Build history of the part. All positions in model axes, mm. Face numbers are marked on the shaded views. A direction names the side the tool comes from. Round coordinates to 2 decimals unless told otherwise and drop trailing zeros. Write each loop counter-clockwise with the first axis right and the second up, starting at its lowest first coordinate (ties: lowest second). Pieces come first, ordered by that corner, then holes. Notation, with made-up numbers: (0, 40) - (51, 40) arc R20 cw to (51, 47) - close; hole circle Ø2 at (-19.75, 87). An arc over 180 degrees is marked (long way). Answer as a JSON object with one key per item and string values. Group by question number.
Item 1: Slice it at A-A, the plane z = 3. List the corners of the cut face in (x, y).
Item 2: Flat gauge pins, fed straight in: pin 1 (6 mm diameter, centred on y = 5.5, z = 1.5, fed in from +X); pin 2 (3.5 mm diameter, centred on x = 6.5, y = 3.5, fed in from -Z); pin 3 (1.6 mm diameter, centred on x = 56.5, y = 6.5, fed in from +Z). Where does each tip first touch, or does it go through?
Item 3: Which spindle directions (+Z, -Z, +X, -X, +Y, -Y) get a long thin tool onto all of the face, cutting with end or side? Do the marked faces 1 and 2. Say none if no direction does.
Item 4: Probe line 1 (X direction, y = 3, z = -25.5); line 2 (X direction, y = 1.75, z = -19.5); line 3 (X direction, y = 6.75, z = -1.5). List the from-to ranges inside material, lowest first. Write a range as from..to.
from build123d import *

# Parameters (mm, degrees)
BOSS_EXTRUDE1_DEPTH = 12.7


with BuildPart() as part:
    # Sketch1 → Boss-Extrude1 (new body)
    with BuildSketch(Plane(origin=(0, 0, 0), x_dir=(1, 0, 0), z_dir=(0, 1, 0))):
        with BuildLine():
            Line((-45.143401222, -37.21280371), (53.277347388, -37.21280371))
            ThreePointArc((53.277347388, -37.21280371), (90.490151098, 0), (53.277347388, 37.21280371))
            Line((53.277347388, 37.21280371), (27.692764767, 37.21280371))
            Line((27.692764767, 37.21280371), (12.941319101, 27.952087025))
            Line((12.941319101, 27.952087025), (8.540643474, 30.705646777))
            Line((8.540643474, 30.705646777), (4.066973083, 30.705646777))
            Line((4.066973083, 30.705646777), (-4.969353988, 16.263997468))
            Line((-4.969353988, 16.263997468), (-12.306945735, 27.952087025))
            Line((-12.306945735, 27.952087025), (-21.201307507, 22.368351957))
            Line((-21.201307507, 22.368351957), (-26.43532504, 30.705646777))
            Line((-26.43532504, 30.705646777), (-26.43532504, 14.031057137))
            Line((-26.43532504, 14.031057137), (-36.903360106, 30.705646777))
            Line((-36.903360106, 30.705646777), (-39.449638906, 24.198489844))
            Line((-39.449638906, 24.198489844), (-45.143401222, 37.21280371))
            ThreePointArc((-45.143401222, 37.21280371), (-74.127657469, 23.338929919), (-81.499787082, -7.937629821))
            Line((-81.499787082, -7.937629821), (-63.784157153, -7.937629821))
            Line((-63.784157153, -7.937629821), (-72.641972118, -11.70947558))
            Line((-72.641972118, -11.70947558), (-68.727071589, -12.511169013))
            Line((-68.727071589, -12.511169013), (-70.684521854, -14.91719786))
            Line((-70.684521854, -14.91719786), (-64.97814292, -14.91719786))
            Line((-64.97814292, -14.91719786), (-68.180229032, -17.32540427))
            Line((-68.180229032, -17.32540427), (-67.831332387, -19.673301397))
            Line((-67.831332387, -19.673301397), (-68.906488172, -20.481898343))
            Line((-68.906488172, -20.481898343), (-64.97814292, -21.037775518))
            Line((-64.97814292, -21.037775518), (-68.906488172, -28.637535833))
            Line((-68.906488172, -28.637535833), (-45.143401222, -37.21280371))
        make_face()
        Polygon((67.312961335, 3.038472361), (73.091855891, 5.285820244), (70.766094983, 0), (75.147452652, 0), (68.896846804, -6.250605848), (68.896846804, -12.511169013), (61.782570481, -9.38088743), (57.594408206, -13.569049705), (59.688489343, 0), (54.402669099, 5.285820244), (59.688489343, 5.285820244), (65.339708642, 10.937039543), align=None, mode=Mode.SUBTRACT)
    extrude(amount=BOSS_EXTRUDE1_DEPTH)


solid = part.part
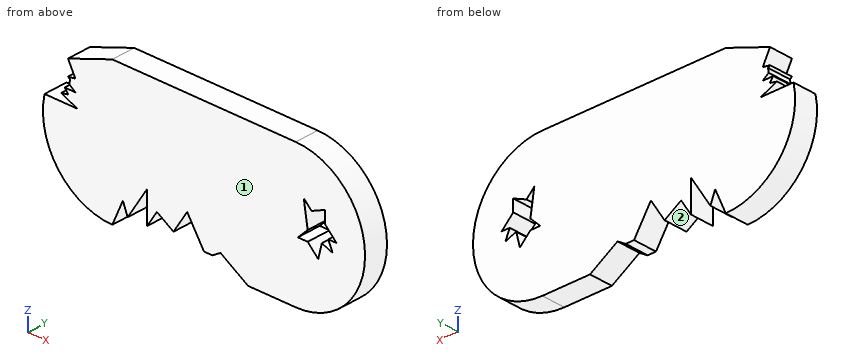
Geometry says:
{
 "1": {"outline": "(-82.24, 0) - (59.23, 0) - (59.23, 12.7) - (-82.24, 12.7) - close; (72.15, 0) - (90.37, 0) - (90.37, 12.7) - (72.15, 12.7) - close"},
 "2": {"pin 1": "stops at x = 90.49", "pin 2": "stops at z = -30.71", "pin 3": "stops at z = 37.13"},
 "3": {"face 1": "+Z, -Z, +X, -X, -Y", "face 2": "-Z, +Y, -Y"},
 "4": {"line 1": "x = -72.25..-40.02, -38.94..-33.64, -26.44..-23.17, -16.21..-10.77, 0.81..80.38", "line 2": "x = -76.84..-29.87, -26.44..-7, -2.94..84.97", "line 3": "x = -82.33..58.19, 71.43..90.46"}
}
